from build123d import *

# Parameters (mm, degrees)
F0_R           = 11.5
F0_R_2         = 10
F1_DEPTH       = 5
F5_DEPTH       = 10
F5_DEPTH_BACK  = 10
F6_W           = 4.5
F6_H           = 2.5
F7_DEPTH       = 0.5
F7_DEPTH_BACK  = 20.5
F8_R           = 3
F9_DEPTH       = 0.5
F9_DEPTH_BACK  = 0.5
F13_DEPTH      = 2.5
F13_DEPTH_BACK = 2.5


with BuildPart() as f1:
    # F0 (on Right) → F1 (new body)
    with BuildSketch(Plane.YZ):
        Circle(F0_R)
        Circle(F0_R_2, mode=Mode.SUBTRACT)
    extrude(amount=F1_DEPTH)


with BuildPart() as f3_1:
    # F3: copy of F1
    add(f1.part.moved(Location((0, 0, 22))))


with BuildPart() as f1_1:
    add(f1.part)

    add(f3_1.part)  # F5 merges F3_1
    # F4 (on offset) → F5 (join, two sides)
    with BuildSketch(Plane(origin=(2.5, 0, 0), x_dir=(0, -1, 0), z_dir=(-1, 0, 0))) as f5_sk:
        with BuildLine():
            Line((-12, 44), (-12, 39))
            Line((-12, 39), (-10, 39))
            ThreePointArc((-10, 39), (-11.1478150705, 41.3704369859), (-11, 44))
            Line((-11, 44), (-12, 44))
        make_face()
        with BuildLine():
            Line((-12, 39), (-12, -16))
            Line((-12, -16), (-8, -16))
            Line((-8, -16), (-8, -14))
            Line((-8, -14), (-8, -8.2613558209))
            ThreePointArc((-8, -8.2613558209), (-11.5, 0), (-8, 8.2613558209))
            Line((-8, 8.2613558209), (-8, 13.7386441791))
            ThreePointArc((-8, 13.7386441791), (-11.5, 22), (-8, 30.2613558209))
            Line((-8, 30.2613558209), (-8, 37))
            Line((-8, 37), (-8, 39))
            Line((-8, 39), (-10, 39))
            Line((-10, 39), (-12, 39))
        make_face()
        with BuildLine():
            ThreePointArc((-8, 30.2613558209), (-11.5, 22), (-8, 13.7386441791))
            Line((-8, 13.7386441791), (-8, 30.2613558209))
        make_face()
        with BuildLine():
            ThreePointArc((-8, 8.2613558209), (-11.5, 0), (-8, -8.2613558209))
            Line((-8, -8.2613558209), (-8, 8.2613558209))
        make_face()
    extrude(amount=F5_DEPTH)
    extrude(f5_sk.sketch, amount=-F5_DEPTH_BACK)

    # F6 (on face) → F7 (join, two sides)
    with BuildSketch(Plane(origin=(-7.5, 0, 0), x_dir=(0, -1, 0), z_dir=(-1, 0, 0))) as f7_sk:
        with Locations((-10.25, 0)):
            Rectangle(F6_W, F6_H)
        with Locations((-10.25, 22)):
            Rectangle(F6_W, F6_H)
    extrude(amount=F7_DEPTH)
    extrude(f7_sk.sketch, amount=-F7_DEPTH_BACK)

    # F8 (on face) → F9 (join, two sides)
    with BuildSketch(Plane(origin=(0, 12.5, 0), x_dir=(-1, 0, 0), z_dir=(0, 1, 0))) as f9_sk:
        with Locations((-2.5, 22)):
            Circle(F8_R)
        with Locations((-2.5, 0)):
            Circle(F8_R)
    extrude(amount=F9_DEPTH)
    extrude(f9_sk.sketch, amount=-F9_DEPTH_BACK)

    # F10 (on offset) → F11 (revolve)
    with BuildSketch(Plane(origin=(2.5, 0, 0), x_dir=(0, -1, 0), z_dir=(-1, 0, 0))):
        Polygon((-13, -2), (-13, 0), (-13.9, 0), (-14.5, -0.3), align=None)
    revolve(axis=Axis((2.5, 13.75, 0), (0, 1, 0)))

    # F10 (on offset) → F12 (revolve)
    with BuildSketch(Plane(origin=(2.5, 0, 0), x_dir=(0, -1, 0), z_dir=(-1, 0, 0))):
        Polygon((-13, 24), (-14.5, 22.3), (-13.9, 22), (-13, 22), align=None)
    revolve(axis=Axis((2.5, 13.75, 22), (0, 1, 0)))

    # F4 (on offset) → F13 (join, two sides)
    with BuildSketch(Plane(origin=(2.5, 0, 0), x_dir=(0, -1, 0), z_dir=(-1, 0, 0))) as f13_sk:
        with BuildLine():
            ThreePointArc((-6, 31.8107084352), (-7.1956056108, 34.3299660424), (-8, 37))
            Line((-8, 37), (-8, 30.2613558209))
            ThreePointArc((-8, 30.2613558209), (-7.0427355041, 31.0911977549), (-6, 31.8107084352))
        make_face()
        with BuildLine():
            Line((-8, -8.2613558209), (-8, -14))
            ThreePointArc((-8, -14), (-7.1707018436, -11.8238598451), (-6, -9.8107084352))
            ThreePointArc((-6, -9.8107084352), (-7.0427355041, -9.0911977549), (-8, -8.2613558209))
        make_face()
    extrude(amount=F13_DEPTH)
    extrude(f13_sk.sketch, amount=-F13_DEPTH_BACK)


solid = f1_1.part
The listing builds one solid part. Answer for the finished solid, in the listing's coordinates (mm). A direction names the side the tool comes from. Coordinates: 2 decimals unless noted, no trailing zeros. Write each loop counter-clockwise with the first axis right and the second up, starting at its lowest first coordinate (ties: lowest second). Pieces come first, ordered by that corner, then holes. Notation, with made-up numbers: (-6.5, 78.5) - (52.5, 78.5) arc R28 ccw to (52.5, 117.5) - close; hole circle Ø4 at (-31.75, -10). An arc over 180 degrees is marked (long way). Answer as CSV lines item,"result".
1. Determine the mould class of faces 4 (the cylindrical face through (2.46, 7.18, 34.29)), 5 (the cylindrical face through (2, -10, 22)), 6 (the cylindrical face through (2.36, 11.14, 41.33)), 7 (the flat face through (2, 10, -16)) for opening direction Z: +Z half, -Z half, draft (parallel to the pull), parting line (faces both ways), or undercut.
Computed values:
face 4,"+Z half"
face 5,"undercut"
face 6,"undercut"
face 7,"-Z half"
2. Find section D-D (x = -1.5). Give the vertices of the cut face in (y, z).
Computed values:
outline,"(8, -16) - (12, -16) - (12, -1.25) - (12.5, -1.25) - (12.5, 1.25) - (12, 1.25) - (12, 20.75) - (12.5, 20.75) - (12.5, 23.25) - (12, 23.25) - (12, 44) - (11, 44) arc R5.25 cw to (10, 39) - (8, 39) - close"
3. Straight lines are drawn through the part: line 1 (Z direction, x = 1.5, y = 0); line 2 (Z direction, x = 3, y = 7); line 3 (Z direction, x = 3, y = 2.5). For each, find the intervals that lie inside material, in ascending order. Write a range as [from, to].
Computed values:
line 1,"z = [-11.5, -10], [10, 12], [32, 33.5]"
line 2,"z = [-11.48, -7.14], [7.14, 9.12], [12.88, 14.86], [29.14, 33.84]"
line 3,"z = [-11.22, -9.68], [9.68, 12.32], [31.68, 33.22]"
4. A tool of negligible diameter and unlimited length cuts with its end or side. For faces 1 (the flat face through (5, 13, 0)), 2 (the flat face through (12.5, 10, 31)), 3 (the flat face through (0, -3, 12)), from which of +Z, -Z, +X, -X, +Y, -Y can it reach the whole face along a straight path? Write none if from no direction.
Computed values:
face 1,"+Y"
face 2,"+Z, +X, +Y, -Y"
face 3,"+Z, -Z, -X, -Y"
5. Find section A-A (y = 0). Give the vertices of the cut face in (x, z), plus the area to 3 significant figures.
Computed values:
outline,"(0, -11.5) - (5, -11.5) - (5, -10) - (0, -10) - close; (0, 10) - (5, 10) - (5, 12) - (0, 12) - close; (0, 32) - (5, 32) - (5, 33.5) - (0, 33.5) - close"
area,"25.0 mm²"
6. Given P1, Ø3, axis at x = -2.5, z = -0.5, coming from the +Y side; P2, Ø2, axis at y = 10.5, z = -9.5, coming from the -X side; P3, Ø4, axis at y = 7, z = 17.5, coming from the +X side; P4, Ø6, axis at y = 3, z = 3.5, coming from the +X side, each flat-ended and moving along its own axis, determine where each tip first touches the part or whether it passes through.
Computed values:
P1,"stops at y = 12.5"
P2,"stops at x = -7.5"
P3,"stops at x = 12.5"
P4,"passes through"
7. Find section B-B (z = 15). Give the vertices of the cut face in (x, y), plus the area to 3 significant figures.
Computed values:
outline,"(-7.5, 8) - (0, 8) - (0, 7.14) - (5, 7.14) - (5, 8) - (12.5, 8) - (12.5, 12) - (-7.5, 12) - close; (0, -9.12) - (5, -9.12) - (5, -7.14) - (0, -7.14) - close"
area,"94.2 mm²"
8. Find section C-C (y = 7). Give the vertices of the cut face in (x, z), plus the area to 3 significant figures.
Computed values:
outline,"(0, -11.48) - (5, -11.48) - (5, -7.14) - (0, -7.14) - close; (0, 7.14) - (5, 7.14) - (5, 9.12) - (0, 9.12) - close; (0, 12.88) - (5, 12.88) - (5, 14.86) - (0, 14.86) - close; (0, 29.14) - (5, 29.14) - (5, 33.84) - (0, 33.84) - close"
area,"65.0 mm²"
